Here's how the part is built. I have some questions about the finished solid (model axes, mm). Face numbers are marked on the shaded views. Give positions to 0.01 mm unless a question says otherwise; leave off trailing zeros. Loops run counter-clockwise (first coordinate to the right, second up) from the corner with the lowest first, then second, coordinate; pieces in that order, holes last. Notation, with made-up numbers: (-27, 37.25) - (-23, 37.25) arc R31 ccw to (-23, 70.25) - close; hole circle Ø4 at (17, 75). An arc over 180 degrees is marked (long way). Use a Markdown table: item, result.
from build123d import *

# Parameters (mm, degrees)
SKETCH_R        = 25
SKETCH_R_2      = 1.5
PAD_DEPTH       = 9
SKETCH002_R     = 3
POCKET_DEPTH    = 28
SKETCH003_R     = 5.1
POCKET001_DEPTH = 1
CHAMFER_SIZE    = 0.6


with BuildPart() as part:
    # Sketch → Pad (new body)
    with BuildSketch(Plane.XY):
        Circle(SKETCH_R)
        with Locations((0, 11)):
            Circle(SKETCH_R_2, mode=Mode.SUBTRACT)
        with Locations((-11, 0)):
            Circle(SKETCH_R_2, mode=Mode.SUBTRACT)
        with Locations((0, -11)):
            Circle(SKETCH_R_2, mode=Mode.SUBTRACT)
        with Locations((11, 0)):
            Circle(SKETCH_R_2, mode=Mode.SUBTRACT)
    extrude(amount=PAD_DEPTH)

    # Sketch002 (on Face7 of Pad) → Pocket (cut)
    with BuildSketch(Plane.XY.offset(9)):
        Circle(SKETCH002_R)
    extrude(amount=-POCKET_DEPTH, mode=Mode.SUBTRACT)

    # Sketch003 (on Face2 of Pocket) → Pocket001 (cut)
    with BuildSketch(Plane(origin=(0, 0, 0), x_dir=(1, 0, 0), z_dir=(0, 0, -1))):
        Circle(SKETCH003_R)
    extrude(amount=-POCKET001_DEPTH, mode=Mode.SUBTRACT)

    # Chamfer
    chamfer_edges = [part.edges().sort_by_distance(p)[0] for p in [
        (-1.5, 11, 0),
        (-25, 0, 0),
        (9.5, 0, 0),
        (-1.5, -11, 0),
        (-12.5, 0, 0),
        (-5.1, 0, 0),
        (-3, 0, 1),
        (9.5, 0, 9),
        (-1.5, 11, 9),
        (-3, 0, 9),
        (-12.5, 0, 9),
        (-1.5, -11, 9),
        (-25, 0, 9),
    ]]
    chamfer(chamfer_edges, length=CHAMFER_SIZE)


solid = part.part
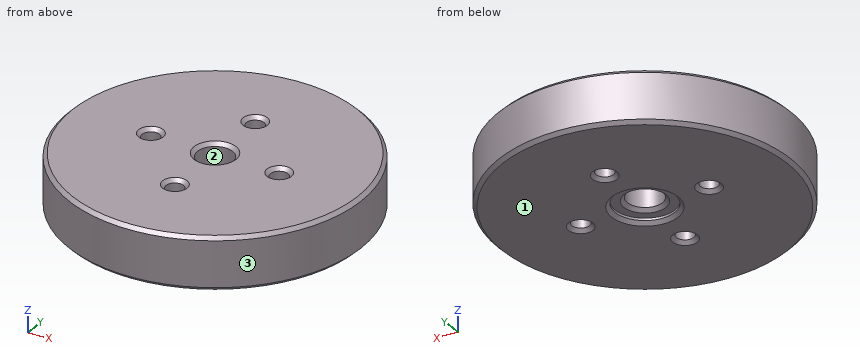
(1) If I drill on line 1 (Y direction, x = 0, z = 0.9); line 2 (Y direction, x = 0, z = 3); line 3 (Y direction, x = 11, z = 4), over which ranges is the centre line in solid material (lowest first)?
A:
| item | result |
|---|---|
| line 1 | -25 to -12.5, -9.5 to -5.1, 5.1 to 9.5, 12.5 to 25 |
| line 2 | -25 to -12.5, -9.5 to -3, 3 to 9.5, 12.5 to 25 |
| line 3 | -22.45 to -1.5, 1.5 to 22.45 |
(2) Will these pins go through, and if not, where does the flat tip stop? pin 1 (3.5 mm diameter, centred on x = -11, y = 0, fed in from +Z); pin 2 (3.5 mm diameter, centred on x = 11, y = 0, fed in from -Z); pin 3 (7 mm diameter, centred on x = 0, y = 0, fed in from -Z).
A:
| item | result |
|---|---|
| pin 1 | z = 8.65 |
| pin 2 | z = 0.35 |
| pin 3 | z = 1.1 |
(3) We'd pull the mould along X, two halves only. Please class the marked faces 1, 2 and 3: pulls with the +X half, pulls with the -X half, needs draft (parallel to the pull), parting line crosses it, or undercut.
A:
| item | result |
|---|---|
| face 1 | needs draft |
| face 2 | undercut |
| face 3 | parting line crosses it |
(4) Suppose I cut it at A-A on x = 0. Count the separate pieces of the cut face and the enclosed holes in it, plus the area to 3 significant figures.
A:
| item | result |
|---|---|
| separate pieces | 4 |
| enclosed holes | 0 |
| area | 335 mm2 |
(5) Suppose I cut it at B-B on z = 2.25. Write out the boundary of the cut face in (x, y), plus the area to 3 significant figures.
A:
| item | result |
|---|---|
| outline | circle Ø50 at (0, 0); hole circle Ø3 at (-11, 0); hole circle Ø6 at (0, 0); hole circle Ø3 at (0, -11); hole circle Ø3 at (0, 11); hole circle Ø3 at (11, 0) |
| area | 1,910 mm2 |
